from build123d import *

# Parameters (mm, degrees)
CHAMFER1_SIZE = 3
CHAMFER2_SIZE = 1


with BuildPart() as part:
    # Sketch1 → Revolve1 (revolve)
    with BuildSketch(Plane.XY, mode=Mode.PRIVATE) as revolve1_sk:
        Polygon((2.5, 40.545486338), (11.269263071, 40.545486338), (11.269263071, 51.545486338), (21.5, 51.545486338), (21.5, 46.045486338), (16, 46.045486338), (16, 35.645486338), (21.5, 35.645486338), (21.5, 30.145486338), (2.5, 30.145486338), align=None)
    revolve(revolve1_sk.sketch.rotate(Axis((0, 0, 0), (0, 1, 0)), 90), axis=Axis((0, 0, 0), (0, 1, 0)))

    # Chamfer1
    chamfer1_edges = [part.edges().sort_by_distance(p)[0] for p in [
        (0, 51.545486338, 11.269263071),
    ]]
    chamfer(chamfer1_edges, length=CHAMFER1_SIZE)

    # Chamfer2
    chamfer2_edges = [part.edges().sort_by_distance(p)[0] for p in [
        (0, 30.145486338, 21.5),
        (0, 51.545486338, 21.5),
    ]]
    chamfer(chamfer2_edges, length=CHAMFER2_SIZE)


solid = part.part
Model file for the job. Use its own axes, mm. A direction names the side the tool comes from. Give positions to 0.01 mm unless a question says otherwise; leave off trailing zeros. Loops run counter-clockwise (first coordinate to the right, second up) from the corner with the lowest first, then second, coordinate; pieces in that order, holes last. Notation, with made-up numbers: (4, -9.75) -> (48, -9.75) arc R29 ccw to (48, 23.25) -> close; hole circle Ø3 at (76, -28.75). An arc over 180 degrees is marked (long way). Use a Markdown table: item, result. Add a question column.
(1) Tool access for faces 1 (the flat face through (-3, 40.545, 0)), 2 (the flat face through (-16, 46.045, 3)), 3 (the flat face through (0, 30.145, -4)): list every direction of +Z, -Z, +X, -X, +Y, -Y with a clear straight run to the whole face (end or side of a thin tool).
(2) Mould opens along Z. For faces 4 (the flat face through (-16, 35.645, -3)), 5 (the cylindrical face through (-21.317, 48.264, 2.799)), 6 (the cylindrical face through (-3.38, 44.6, -10.75)), 7 (the cylindrical face through (-0.1, 35.4, 2.5)) say: +Z half, -Z half, draft (parallel to the pull), parting line (faces both ways), or undercut.
(3) Wall check: line 1 along Y through (x, z) = (7, -16); line 2 along X through (y, z) = (42.75, 0); line 3 along X through (y, z) = (35.25, 0). Give the ranges that are in metal, low to high.
(4) Slice it at C-C on y = 37.75. List the corners of the cut face in (x, z), and give its area (3 significant figures).
(5) Slice it at A-A on z = 0. List the corners of the cut face in (x, y).
(6) Slice it at B-B on x = 0. List the corners of the cut face in (y, z), and give its area (3 significant figures).
(7) Drop flat-ended pins along their axis: pin 1 Ø12 at (y, z) = (32.5, -14) entering from +X; pin 2 Ø3 at (y, z) = (46, 9) entering from -X; pin 3 Ø6 at (y, z) = (34.5, 8) entering from -X. Give the stop position or say it passes through.
Filled sheet:
| question | item | result |
|---|---|---|
| 1 | face 1 | +Y |
| 1 | face 2 | none |
| 1 | face 3 | +Z, -Z, +X, -X, -Y |
| 2 | face 4 | draft |
| 2 | face 5 | parting line |
| 2 | face 6 | undercut |
| 2 | face 7 | undercut |
| 3 | line 1 | 30.15 to 35.65, 46.05 to 51.55 |
| 3 | line 2 | -16 to -11.27, 11.27 to 16 |
| 3 | line 3 | -21.5 to -2.5, 2.5 to 21.5 |
| 4 | outline | circle Ø32 at (0, 0); hole circle Ø5 at (0, 0) |
| 4 | area | 785 mm2 |
| 5 | outline | (-21.5, 31.15) -> (-20.5, 30.15) -> (-2.5, 30.15) -> (-2.5, 40.55) -> (-11.27, 40.55) -> (-11.27, 48.55) -> (-14.27, 51.55) -> (-20.5, 51.55) -> (-21.5, 50.55) -> (-21.5, 46.05) -> (-16, 46.05) -> (-16, 35.65) -> (-21.5, 35.65) -> close; (2.5, 30.15) -> (20.5, 30.15) -> (21.5, 31.15) -> (21.5, 35.65) -> (16, 35.65) -> (16, 46.05) -> (21.5, 46.05) -> (21.5, 50.55) -> (20.5, 51.55) -> (14.27, 51.55) -> (11.27, 48.55) -> (11.27, 40.55) -> (2.5, 40.55) -> close |
| 6 | outline | (30.15, -20.5) -> (31.15, -21.5) -> (35.65, -21.5) -> (35.65, -16) -> (46.05, -16) -> (46.05, -21.5) -> (50.55, -21.5) -> (51.55, -20.5) -> (51.55, -14.27) -> (48.55, -11.27) -> (40.55, -11.27) -> (40.55, -2.5) -> (30.15, -2.5) -> close; (30.15, 2.5) -> (40.55, 2.5) -> (40.55, 11.27) -> (48.55, 11.27) -> (51.55, 14.27) -> (51.55, 20.5) -> (50.55, 21.5) -> (46.05, 21.5) -> (46.05, 16) -> (35.65, 16) -> (35.65, 21.5) -> (31.15, 21.5) -> (30.15, 20.5) -> close |
| 6 | area | 495 mm2 |
| 7 | pin 1 | x = 19.96 |
| 7 | pin 2 | x = -20.15 |
| 7 | pin 3 | x = -20.91 |
